Work out the finished part from the listing and answer in its coordinate system (mm). A direction names the side the tool comes from. Coordinates: 2 decimals unless noted, no trailing zeros. Order: outer loops, then holes, each group sorted by start corner. A loop starts at its lowest first (then second) coordinate and runs counter-clockwise, first axis right, second up. Notation, with made-up numbers: M -40,53 L -11,53 A29 ccw -11,92 Z; hole C -37.5,81.25 d5. An arc over 180 degrees is marked long. Answer in a Markdown table with one row per item. Add a question column.
Item 1: Consider line 1 (Z direction, x = -18, y = 29.25); line 2 (X direction, y = 27.75, z = 4.5); line 3 (X direction, y = 30, z = 5.5). Determine where each line is inside the solid, lowest interval first. Write a range as from..to.
Item 2: Which of the six approach directions +Z, -Z, +X, -X, +Y, -Y give full straight-line access (tool end or side, diameter ignored) to faces 1 (the face through (-13.52, 33.6, 4.77)), 2 (the face through (-18.419, 22.945, 4.684))?
Item 3: The part is cut by section B-B (y = 11.25). Write down the section's boundary in (x, z), then the cut area to 3 significant figures.
Item 4: The part is cut by section C-C (y = 31.5). State how many separate pieces and enclosed holes the cut face has, then the cut area to 3 significant figures.
Item 5: The part is cut by section A-A (z = 7.75). Write down the section's boundary in (x, y).
Item 6: The mould has two halves that part along Z. Classify faces 3 (the face through (0, 25, 9.5)), 4 (the face through (18.037, 22.562, 4.684)), 5 (the face through (13.52, 33.6, 4.77)), 6 (the face through (0, 25, 0)): released by +Z, released by -Z, zero draft, split by the parting line, or undercut.
Item 7: Flat-ended cylindrical pins translate along their axes: pin 1 Ø5 at (x, y) = (-23, 31) entering from -Z; pin 2 Ø1.5 at (x, z) = (-25, 3) entering from -Y. Find the tip coordinate at first contact, or state that the pin passes through.
from build123d import *

# Parameters (mm, degrees)
BOSS_EXTRUDE1_DEPTH = 9.5
SKETCH5_R           = 1.5
CUT_EXTRUDE3_DEPTH  = 11


with BuildPart() as part:
    # Sketch1 → Boss-Extrude1 (new body)
    with BuildSketch(Plane.XY):
        with BuildLine():
            Line((4.565685425, 9.091168825), (31.890515832, 36.415999231))
            Line((31.890515832, 36.415999231), (-31.890515832, 36.415999231))
            Line((-31.890515832, 36.415999231), (-4.565685425, 9.091168825))
            ThreePointArc((-4.565685425, 9.091168825), (0, 7.2), (4.565685425, 9.091168825))
        make_face()
    extrude(amount=BOSS_EXTRUDE1_DEPTH)

    # Sketch5 → Cut-Extrude3 (cut)
    with BuildSketch(Plane(origin=(2.2627417, 2.2627417, 0), x_dir=(0, 0, 1), z_dir=(-0.7071067811865512, -0.7071067811865438, 0))):
        with Locations(Location((4.75, 33.3, 0), (0, 0, 270))):
            Circle(SKETCH5_R)
        with Locations(Location((4.75, 18.3, 0), (0, 0, 270))):
            Circle(SKETCH5_R)
    cut_extrude3 = extrude(amount=-CUT_EXTRUDE3_DEPTH, mode=Mode.SUBTRACT)

    # Mirror1: Cut-Extrude3 across plane
    add(cut_extrude3.mirror(Plane(origin=(0, 0, 0), x_dir=(0, 0, 1), z_dir=(1, 0, 0))), mode=Mode.SUBTRACT)


solid = part.part
Reply:
| question | item | result |
|---|---|---|
| 1 | line 1 | z = 0..3.25, 6.25..9.5 |
| 1 | line 2 | x = -23.22..-21.43, -17.25..17.25, 21.43..23.22 |
| 1 | line 3 | x = -25.47..-18.93, -15.26..15.26, 18.93..25.47 |
| 2 | face 1 | none |
| 2 | face 2 | +Z, -Z, -X, -Y |
| 3 | outline | M -6.72,0 L 6.72,0 L 6.72,9.5 L -6.72,9.5 Z |
| 3 | area | 128 mm2 |
| 4 | separate pieces | 1 |
| 4 | enclosed holes | 2 |
| 4 | area | 493 mm2 |
| 5 | outline | M -31.89,36.42 L -4.57,9.09 A6.46 ccw 4.57,9.09 L 31.89,36.42 Z |
| 6 | face 3 | released by +Z |
| 6 | face 4 | zero draft |
| 6 | face 5 | undercut |
| 6 | face 6 | released by -Z |
| 7 | pin 1 | stops at z = 0 |
| 7 | pin 2 | stops at y = 28.78 |
